Geometry check sheet. Reference: the model listing, model coordinates, mm. A direction names the side the tool comes from. Coordinates: 2 decimals unless noted, no trailing zeros. Loops run counter-clockwise (first coordinate to the right, second up) from the corner with the lowest first, then second, coordinate; pieces in that order, holes last.
from build123d import *

# Parameters (mm, degrees)
SKETCH_1_R          = 6.75
EXTRUDE_1_DEPTH     = 1.8
SKETCH_2_R          = 0.8
CUT_EXTRUDE_1_DEPTH = 2
SKETCH_3_R          = 1.75
CUT_EXTRUDE_2_DEPTH = 0.5
CUT_EXTRUDE_4_DEPTH = 10
SKETCH_6_R          = 1.75
EXTRUDE_2_DEPTH     = 1.8


with BuildPart() as part:
    # 草图1 → 凸台-拉伸1 (new body)
    with BuildSketch(Plane.XY):
        with BuildLine():
            Line((0.7, 0), (19.5, 0))
            ThreePointArc((19.5, 0), (19.994974747, -0.205025253), (20.2, -0.7))
            Line((20.2, -0.7), (20.2, -39.6))
            ThreePointArc((20.2, -39.6), (19.994974747, -40.094974747), (19.5, -40.3))
            Line((19.5, -40.3), (0.7, -40.3))
            ThreePointArc((0.7, -40.3), (0.205025253, -40.094974747), (0, -39.6))
            Line((0, -39.6), (0, -0.7))
            ThreePointArc((0, -0.7), (0.205025253, -0.205025253), (0.7, 0))
        make_face()
        with Locations((10.1, -10.1)):
            Circle(SKETCH_1_R, mode=Mode.SUBTRACT)
    extrude(amount=EXTRUDE_1_DEPTH)

    # 草图2 → 切除-拉伸1 (cut)
    with BuildSketch(Plane.XY.offset(1.8)):
        with Locations((17.6, -2.6)):
            Circle(SKETCH_2_R)
        with Locations((17.6, -37.6)):
            Circle(SKETCH_2_R)
        with Locations((2.6, -37.6)):
            Circle(SKETCH_2_R)
        with Locations((2.6, -2.6)):
            Circle(SKETCH_2_R)
    extrude(amount=-CUT_EXTRUDE_1_DEPTH, mode=Mode.SUBTRACT)

    # 草图3 → 切除-拉伸2 (cut)
    with BuildSketch(Plane(origin=(0, 0, 0), x_dir=(-1, 0, 0), z_dir=(0, 0, -1))):
        with Locations((-17.6, -2.6)):
            Circle(SKETCH_3_R)
        with Locations((-2.6, -2.6)):
            Circle(SKETCH_3_R)
        with Locations((-17.6, -37.6)):
            Circle(SKETCH_3_R)
        with Locations((-2.6, -37.6)):
            Circle(SKETCH_3_R)
    extrude(amount=-CUT_EXTRUDE_2_DEPTH, mode=Mode.SUBTRACT)

    # 草图4 → 切除-拉伸4 (cut)
    with BuildSketch(Plane(origin=(0, 0, 0), x_dir=(-1, 0, 0), z_dir=(0, 0, -1))):
        with BuildLine():
            Line((-19.5, -40.3), (-0.7, -40.3))
            ThreePointArc((-0.7, -40.3), (-0.205025253, -40.094974747), (0, -39.6))
            Line((0, -39.6), (0, -0.7))
            ThreePointArc((0, -0.7), (-0.205025253, -0.205025253), (-0.7, 0))
            Line((-0.7, 0), (-19.5, 0))
            ThreePointArc((-19.5, 0), (-19.994974747, -0.205025253), (-20.2, -0.7))
            Line((-20.2, -0.7), (-20.2, -39.6))
            ThreePointArc((-20.2, -39.6), (-19.994974747, -40.094974747), (-19.5, -40.3))
        make_face()
        with BuildLine():
            Line((-0.7, -0.1), (-19.5, -0.1))
            ThreePointArc((-19.5, -0.1), (-19.924264069, -0.275735931), (-20.1, -0.7))
            Line((-20.1, -0.7), (-20.1, -39.6))
            ThreePointArc((-20.1, -39.6), (-19.924264069, -40.024264069), (-19.5, -40.2))
            Line((-19.5, -40.2), (-0.7, -40.2))
            ThreePointArc((-0.7, -40.2), (-0.275735931, -40.024264069), (-0.1, -39.6))
            Line((-0.1, -39.6), (-0.1, -0.7))
            ThreePointArc((-0.1, -0.7), (-0.275735931, -0.275735931), (-0.7, -0.1))
        make_face(mode=Mode.SUBTRACT)
    extrude(amount=-CUT_EXTRUDE_4_DEPTH, mode=Mode.SUBTRACT)

    # 草图6 → 凸台-拉伸2 (add)
    with BuildSketch(Plane(origin=(0, 0, 0), x_dir=(-1, 0, 0), z_dir=(0, 0, -1))):
        with Locations((-17.6, -2.6)):
            Circle(SKETCH_6_R)
        with Locations((-2.6, -2.6)):
            Circle(SKETCH_6_R)
    extrude(amount=-EXTRUDE_2_DEPTH)


solid = part.part
1) Section check B-B on x = 10.1. Record the cut outline in (y, z).
Data:
outline: (-40.2, 0) - (-16.85, 0) - (-16.85, 1.8) - (-40.2, 1.8) - close; (-3.35, 0) - (-0.1, 0) - (-0.1, 1.8) - (-3.35, 1.8) - close
2) Access from +Z, -Z, +X, -X, +Y, -Y to the whole of each face (thin tool, end or side, straight path). Record for faces 4 (the flat face through (10, -40.2, 1)), 5 (the cylindrical face through (19.35, -37.52, 0.25)).
Data:
face 4: +Z, -Z, +X, -X, -Y
face 5: -Z
3) Depth check by flat-ended pin: pin 1 (12 mm diameter, centred on x = 10.1, y = -10.1, fed in from -Z); pin 2 (1 mm diameter, centred on x = 18, y = -37.5, fed in from -Z). Enter the tip coordinate at first touch or a pass-through.
Data:
pin 1: passes through
pin 2: stops at z = 0.5
4) Mould release check, pull along X, two halves, no side actions. Record for faces 1 (the cylindrical face through (17.496, -36.807, 1.159)), 2 (the flat face through (10, -20, 1.8)), 3 (the flat face through (20.1, -20, 1)): +X half, -X half, draft (parallel to the pull), parting line (faces both ways), or undercut.
Data:
face 1: undercut
face 2: draft
face 3: +X half
5) Section check C-C on z = 0.9. Record the cut outline in (x, y).
Data:
outline: (0.1, -39.6) arc R0.6 ccw to (0.7, -40.2) - (19.5, -40.2) arc R0.6 ccw to (20.1, -39.6) - (20.1, -0.7) arc R0.6 ccw to (19.5, -0.1) - (0.7, -0.1) arc R0.6 ccw to (0.1, -0.7) - close; hole circle Ø1.6 at (2.6, -37.6); hole circle Ø13.5 at (10.1, -10.1); hole circle Ø1.6 at (17.6, -37.6)
6) Material ranges on probe 1 along X at (y, z) = (-37.6, 1.1); probe 2 along Y at (x, z) = (2.6, 1.4); probe 3 along X at (y, z) = (-11.5, 0.65), recorded low to high.
Data:
probe 1: x = 0.1 to 1.8, 3.4 to 16.8, 18.4 to 20.1
probe 2: y = -40.2 to -38.4, -36.8 to -0.1
probe 3: x = 0.1 to 3.5, 16.7 to 20.1
7) Section check D-D on y = -37.6. Record the cut outline in (x, z), and give its area (3 significant figures).
Data:
outline: (0.1, 0) - (0.85, 0) - (0.85, 0.5) - (1.8, 0.5) - (1.8, 1.8) - (0.1, 1.8) - close; (3.4, 0.5) - (4.35, 0.5) - (4.35, 0) - (15.85, 0) - (15.85, 0.5) - (16.8, 0.5) - (16.8, 1.8) - (3.4, 1.8) - close; (18.4, 0.5) - (19.35, 0.5) - (19.35, 0) - (20.1, 0) - (20.1, 1.8) - (18.4, 1.8) - close
area: 28.3 mm2
8) Section check A-A on y = -10.1. Record the cut outline in (x, z), and give its area (3 significant figures).
Data:
outline: (0.1, 0) - (3.35, 0) - (3.35, 1.8) - (0.1, 1.8) - close; (16.85, 0) - (20.1, 0) - (20.1, 1.8) - (16.85, 1.8) - close
area: 11.7 mm2
